from build123d import *

# Parameters (mm, degrees)
SKETCH_4_R          = 2.9
EXTRUDE_1_DEPTH     = 34
SKETCH_4_5_R        = 0.7
CUT_EXTRUDE_1_DEPTH = 3
CUT_EXTRUDE_START   = 31
SKETCH_4_6_R        = 0.7
CUT_EXTRUDE_2_DEPTH = 3


with BuildPart() as part:
    # 草图4 → 凸台-拉伸1 (new body)
    with BuildSketch(Plane(origin=(0, 0, 0), x_dir=(1, 0, 0), z_dir=(0, 1, 0))):
        with Locations(Location((0, 0, 0), (0, 0, 270))):
            Circle(SKETCH_4_R)
    extrude(amount=EXTRUDE_1_DEPTH)

    # 草图4<5> → 切除-拉伸1 (cut)
    with BuildSketch(Plane(origin=(0, 0, 0), x_dir=(1, 0, 0), z_dir=(0, 1, 0))):
        with Locations(Location((0, 0, 0), (0, 0, 270))):
            Circle(SKETCH_4_5_R)
    extrude(amount=CUT_EXTRUDE_1_DEPTH, mode=Mode.SUBTRACT)

    # 草图4<6> → 切除-拉伸2 (cut)
    with BuildSketch(Plane(origin=(0, 0, 0), x_dir=(1, 0, 0), z_dir=(0, 1, 0)).offset(CUT_EXTRUDE_START)):
        with Locations(Location((0, 0, 0), (0, 0, 270))):
            Circle(SKETCH_4_6_R)
    extrude(amount=CUT_EXTRUDE_2_DEPTH, mode=Mode.SUBTRACT)


solid = part.part
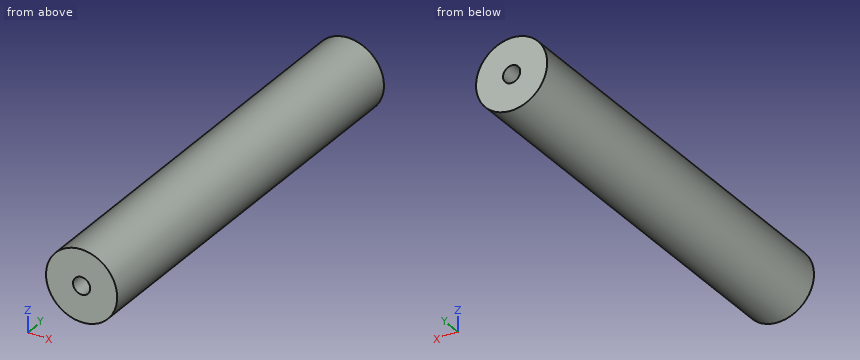
Here's how the part is built. I have some questions about the finished solid (model axes, mm). Round coordinates to 2 decimals unless told otherwise and drop trailing zeros. Loops run counter-clockwise (first coordinate to the right, second up) from the corner with the lowest first, then second, coordinate; pieces in that order, holes last. Notation, with made-up numbers: M -36.5,-37.75 L -4.5,-37.75 A13 cw -4.5,-13.75 Z; hole C -15,-37.75 d6. An arc over 180 degrees is marked long. Write each question's results on one line, items separated by ' | '. Start each with the question number.
(1) I want a section at B-B (x = 0). Please give me the cut outline in (y, z).
(2) I want a section at A-A (z = 0). Please give me the cut outline in (x, y).
(3) I want a section at D-D (x = -1.4). Please give me the cut outline in (y, z), then the cut area to 3 significant figures.
(4) If I drill on probe 1 along X at (y, z) = (1.15, 0); probe 2 along Y at (x, z) = (-0.3, -0.6); probe 3 along Z at (x, y) = (-2.45, 3), over which ranges is the centre line in solid material (lowest first)? Write a range as from..to.
(5) I want a section at C-C (y = 30.5). Please give me the cut outline in (x, z).
(6) Will this pin go through, and if not, where does the flat tip stop? P1, Ø1.1, axis at x = 0, z = 0, coming from the -Y side.
Solved:
1) outline: M 0,-2.9 L 34,-2.9 L 34,-0.7 L 31,-0.7 L 31,0.7 L 34,0.7 L 34,2.9 L 0,2.9 L 0,0.7 L 3,0.7 L 3,-0.7 L 0,-0.7 Z
2) outline: M -2.9,0 L -0.7,0 L -0.7,3 L 0.7,3 L 0.7,0 L 2.9,0 L 2.9,34 L 0.7,34 L 0.7,31 L -0.7,31 L -0.7,34 L -2.9,34 Z
3) outline: M 0,-2.54 L 34,-2.54 L 34,2.54 L 0,2.54 Z | area: 173 mm²
4) probe 1: x = -2.9..-0.7, 0.7..2.9 | probe 2: y = 3..31 | probe 3: z = -1.55..1.55
5) outline: C 0,0 d5.8
6) P1: stops at y = 3
